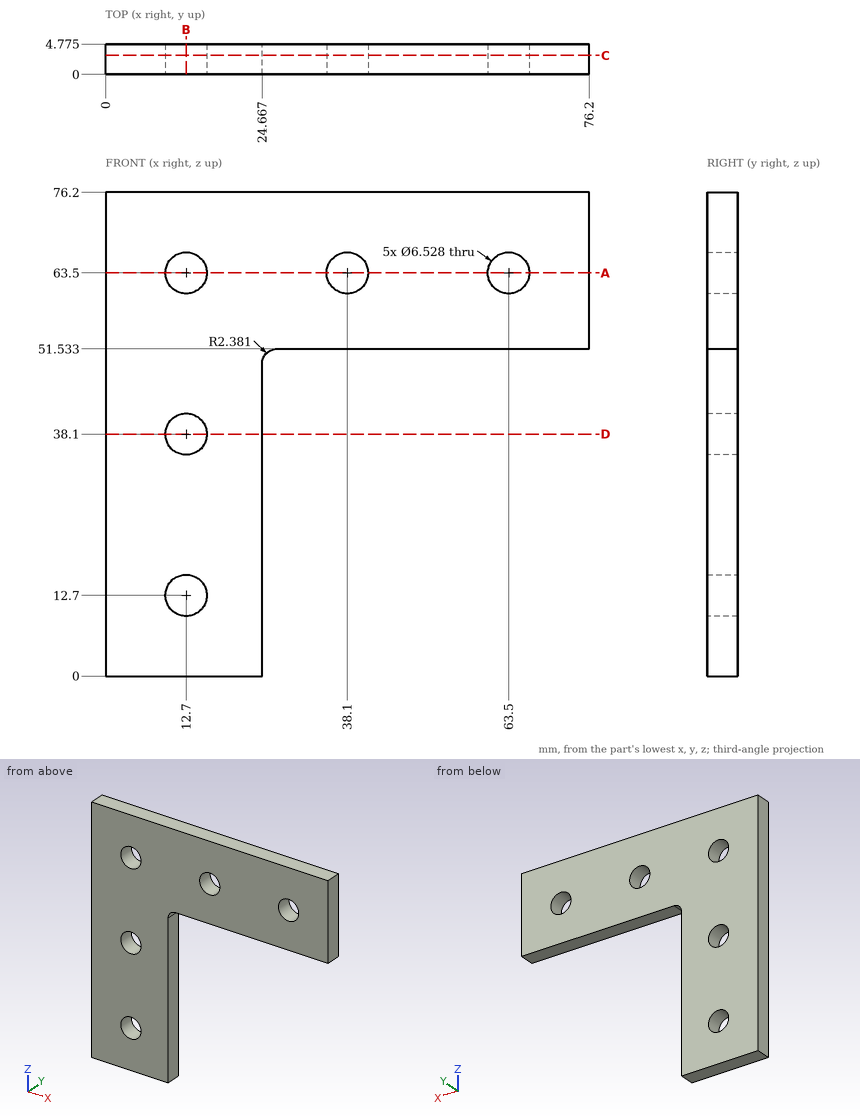
Drawing for the job (mm, zero at the part's lowest x, y, z). Round coordinates to 2 decimals unless told otherwise and drop trailing zeros. Write each loop counter-clockwise with the first axis right and the second up, starting at its lowest first coordinate (ties: lowest second). Pieces come first, ordered by that corner, then holes. Notation, with made-up numbers: (17.5, -14) - (57.5, -14) arc R20 cw to (57.5, -10) - close; hole circle Ø10 at (-18, 28.5). An arc over 180 degrees is marked (long way). Write item = value, one per line. Start each with the question number.
Q1. Band-saw the part on D-D (z = 38.1). Give the cut face in (x, y) (1 decimal), then the cut area to 3 significant figures.
Q2. Band-saw the part on B-B (x = 12.7). Give the cut face in (y, z) (1 decimal).
Q3. Drop flat-ended pins along their axis: pin 1 (1.4 mm diameter, centred on x = 53.5, y = 2, fed in from -Z); pin 2 (1.4 mm diameter, centred on y = 1.5, z = 34, fed in from +X). Give the stop position or say it passes through.
Q4. Band-saw the part on C-C (y = 3). Give the cut face in (x, z), then the cut area to 3 significant figures.
Q5. Band-saw the part on A-A (z = 63.5). Give the cut face in (x, y) (1 decimal), then the cut area to 3 significant figures.
Q6. Probe L1, parallel to X at y = 2.4, z = 63.5; L2, parallel to X at y = 2.7, z = 38.1. List the from-to ranges inside material, lowest first. Write a range as from..to.
Answers below:
q1.outline = (0, 0) - (9.4, 0) - (9.4, 4.8) - (0, 4.8) - close; (16, 0) - (24.7, 0) - (24.7, 4.8) - (16, 4.8) - close
q1.area = 86.6 mm2
q2.outline = (0, 0) - (4.8, 0) - (4.8, 9.4) - (0, 9.4) - close; (0, 16) - (4.8, 16) - (4.8, 34.8) - (0, 34.8) - close; (0, 41.4) - (4.8, 41.4) - (4.8, 60.2) - (0, 60.2) - close; (0, 66.8) - (4.8, 66.8) - (4.8, 76.2) - (0, 76.2) - close
q3.pin_1 = 51.53
q3.pin_2 = 24.67
q4.outline = (0, 0) - (24.67, 0) - (24.67, 49.15) arc R2.38 cw to (27.05, 51.53) - (76.2, 51.53) - (76.2, 76.2) - (0, 76.2) - close; hole circle Ø6.53 at (12.7, 12.7); hole circle Ø6.53 at (12.7, 38.1); hole circle Ø6.53 at (12.7, 63.5); hole circle Ø6.53 at (38.1, 63.5); hole circle Ø6.53 at (63.5, 63.5)
q4.area = 2,980 mm2
q5.outline = (0, 0) - (9.4, 0) - (9.4, 4.8) - (0, 4.8) - close; (16, 0) - (34.8, 0) - (34.8, 4.8) - (16, 4.8) - close; (41.4, 0) - (60.2, 0) - (60.2, 4.8) - (41.4, 4.8) - close; (66.8, 0) - (76.2, 0) - (76.2, 4.8) - (66.8, 4.8) - close
q5.area = 270 mm2
q6.L1 = 0..9.44, 15.96..34.84, 41.36..60.24, 66.76..76.2
q6.L2 = 0..9.44, 15.96..24.67
